from build123d import *

# Parameters (mm, degrees)
SKETCH1_W                = 50
SKETCH1_H                = 50
BOSS_EXTRUDE1_DEPTH      = 25
CHAMFER1_SIZE            = 1.5
BOSS_EXTRUDE2_DEPTH      = 7
BOSS_EXTRUDE2_DEPTH_BACK = 10
SKETCH2_W                = 7
SKETCH2_H                = 1
SKETCH3_W                = 1.8
SKETCH3_H                = 1.8
CUT_EXTRUDE1_DEPTH       = 7


with BuildPart() as part:
    # Sketch1 → Boss-Extrude1 (new body)
    with BuildSketch(Plane.XY):
        with Locations((25, 25)):
            Rectangle(SKETCH1_W, SKETCH1_H)
    extrude(amount=BOSS_EXTRUDE1_DEPTH)

    # Chamfer1
    chamfer1_edges = [part.edges().sort_by_distance(p)[0] for p in [
        (50, 25, 25),
        (25, 50, 25),
        (0, 25, 25),
        (25, 50, 0),
        (50, 25, 0),
        (25, 0, 0),
        (0, 25, 0),
        (25, 0, 25),
        (0, 50, 12.5),
        (50, 50, 12.5),
        (50, 0, 12.5),
        (0, 0, 12.5),
    ]]
    chamfer(chamfer1_edges, length=CHAMFER1_SIZE)

    # Sketch2 → Boss-Extrude2 (add, two sides: drawn at the far end of the back side and taken through both)
    with BuildSketch(Plane.XY.offset(25).offset(-BOSS_EXTRUDE2_DEPTH_BACK)):
        with Locations((25, 49.5)):
            Rectangle(SKETCH2_W, SKETCH2_H)
    extrude(amount=BOSS_EXTRUDE2_DEPTH + BOSS_EXTRUDE2_DEPTH_BACK)

    # Sketch3 → Cut-Extrude1 (cut)
    with BuildSketch(Plane.XZ.offset(-49)):
        with Locations((25, 28.6)):
            Rectangle(SKETCH3_W, SKETCH3_H)
    extrude(amount=-CUT_EXTRUDE1_DEPTH, mode=Mode.SUBTRACT)


solid = part.part
The listing builds one solid part. Answer for the finished solid, in the listing's coordinates (mm). Round coordinates to 2 decimals unless told otherwise and drop trailing zeros. Write each loop counter-clockwise with the first axis right and the second up, starting at its lowest first coordinate (ties: lowest second). Pieces come first, ordered by that corner, then holes. Notation, with made-up numbers: (39.25, 39) - (76.25, 39) arc R27 ccw to (76.25, 76) - close; hole circle Ø1 at (-26.5, 42). An arc over 180 degrees is marked (long way). Use a Markdown table: item, result. Add a question column.
1. For a pull along Y with two mould halves and no side action, classify faces 1 (the face through (0.8, 24.7, 24.3)), 2 (the face through (0.8, 0.7, 12.3)), 3 (the face through (0.8, 49.3, 12.3)) as +Y half, -Y half, draft (parallel to the pull), parting line (faces both ways), or undercut.
2. Consider line 1 (Z direction, x = 17.5, y = 46.5). Determine where the line is inside the solid, lowest interval first.
3. The part is cut by section B-B (x = 43.5). Write down the section's boundary in (y, z).
4. The part is cut by section A-A (x = 25). Write down the section's boundary in (y, z).
5. Flat-ended cylindrical pins translate along their axes: P1, Ø0.8, axis at y = 49.5, z = 28.5, coming from the +X side; P2, Ø23.5, axis at x = 13.5, y = 33, coming from the +Z side; P3, Ø0.8, axis at y = 49.5, z = 26, coming from the -X side. Find the tip coordinate at first contact, or state that the pin passes through.
Reported:
| question | item | result |
|---|---|---|
| 1 | face 1 | draft |
| 1 | face 2 | -Y half |
| 1 | face 3 | +Y half |
| 2 | line 1 | 0 to 25 |
| 3 | outline | (0, 1.5) - (1.5, 0) - (48.5, 0) - (50, 1.5) - (50, 23.5) - (48.5, 25) - (1.5, 25) - (0, 23.5) - close |
| 4 | outline | (0, 1.5) - (1.5, 0) - (48.5, 0) - (50, 1.5) - (50, 27.7) - (49, 27.7) - (49, 24.5) - (48.5, 25) - (1.5, 25) - (0, 23.5) - close; (49, 29.5) - (50, 29.5) - (50, 32) - (49, 32) - close |
| 5 | P1 | x = 28.5 |
| 5 | P2 | z = 25 |
| 5 | P3 | x = 21.5 |
